Read the model definition and answer for the solid it produces. Units are mm, in the model's axes. A direction names the side the tool comes from. Coordinates: 2 decimals unless noted, no trailing zeros. Order: outer loops, then holes, each group sorted by start corner. A loop starts at its lowest first (then second) coordinate and runs counter-clockwise, first axis right, second up. Notation, with made-up numbers: (6, 84.5) - (14, 84.5) arc R27 ccw to (14, 122.5) - close; hole circle Ø4 at (75.25, 56.25). An arc over 180 degrees is marked (long way). Write item = value, one per line.
from build123d import *

# Parameters (mm, degrees)
CUT_EXTRUDE_1_DEPTH      = 170.966173207
CUT_EXTRUDE_1_DEPTH_BACK = 33


with BuildPart() as part:
    # 草图1 → 旋转1 (revolve)
    with BuildSketch(Plane(origin=(0, 0, 0), x_dir=(0, 0, -1), z_dir=(1, 0, 0)), mode=Mode.PRIVATE) as revolve_1_sk:
        with BuildLine():
            Line((-34.6, 0), (-34.6, 35))
            Line((-34.6, 35), (-22, 50))
            Line((-22, 50), (-22, 70))
            Line((-22, 70), (-21, 70))
            Line((-21, 70), (-21, 76))
            ThreePointArc((-21, 76), (0, 86.5), (21, 76))
            Line((21, 76), (21, 70))
            Line((21, 70), (22, 70))
            Line((22, 70), (22, 50))
            Line((22, 50), (34.6, 35))
            Line((34.6, 35), (34.6, 25))
            Line((34.6, 25), (40.4, 19.2))
            Line((40.4, 19.2), (40.4, 12))
            Line((40.4, 12), (45.4, 12))
            Line((45.4, 12), (45.4, 14))
            Line((45.4, 14), (48.4, 14))
            Line((48.4, 14), (48.4, 16))
            Line((48.4, 16), (50.4, 16))
            Line((50.4, 16), (50.4, 8))
            Line((50.4, 8), (83.4, 8))
            Line((83.4, 8), (83.4, 1.5))
            Line((83.4, 1.5), (88.4, 1.5))
            Line((88.4, 1.5), (88.4, 0))
            Line((88.4, 0), (-34.6, 0))
        make_face()
    revolve(revolve_1_sk.sketch.rotate(Axis((0, 0, 0), (0, 0, -1)), 90), axis=Axis((0, 0, 0), (0, 0, -1)))

    # 草图2 → 切除-拉伸1 (cut, two sides: drawn at the far end of the back side and taken through both)
    with BuildSketch(Plane(origin=(0, 0, -83.4), x_dir=(-1, 0, 0), z_dir=(0, 0, -1)).offset(-CUT_EXTRUDE_1_DEPTH_BACK)):
        with BuildLine():
            Line((-5.291502622, 6), (5.291502622, 6))
            ThreePointArc((5.291502622, 6), (0, 8), (-5.291502622, 6))
        make_face()
        with BuildLine():
            Line((-5.291502622, -6), (5.291502622, -6))
            ThreePointArc((5.291502622, -6), (0, -8), (-5.291502622, -6))
        make_face()
    extrude(amount=CUT_EXTRUDE_1_DEPTH + CUT_EXTRUDE_1_DEPTH_BACK, mode=Mode.SUBTRACT)


solid = part.part
1) The part is cut by section A-A (z = -7). Determine the outline of the cut face in (x, y), and give its area (3 significant figures).
Returned:
outline = circle Ø171.1 at (0, 0)
area = 23,000 mm^2
2) For faces 1 (the face through (8, 0, -67)), 2 (the face through (-15.175, 68.335, -21.507)), 3 (the face through (6.3, -10.4, -45.4)), 4 (the face through (0, 6, -67)), 5 (the face through (48, -17, 22)), determine the directions among +Z, -Z, +X, -X, +Y, -Y from which every point of the face is accessible in a straight line to the end or side of a thin tool.
Returned:
face_1 = -Z, +X
face_2 = -Z
face_3 = none
face_4 = -Z, +X, -X, +Y
face_5 = +Z
3) Determine the mould class of faces 6 (the face through (-8, 0, -67)), 7 (the face through (33, 62, -21)), 8 (the face through (0, 13, -40.4)) for opening direction Z: pulls with the +Z half, pulls with the -Z half, needs draft (parallel to the pull), parting line crosses it, or undercut.
Returned:
face_6 = needs draft
face_7 = pulls with the -Z half
face_8 = undercut
4) Flat-ended cylindrical pins translate along their axes: pin 1 Ø11.5 at (x, z) = (-2.5, -69) entering from -Y; pin 2 Ø2 at (y, z) = (-13.5, -7.5) entering from -X; pin 3 Ø6 at (x, z) = (-44.5, 7) entering from -Y. Find the tip coordinate at first contact, or state that the pin passes through.
Returned:
pin_1 = -6
pin_2 = -84.66
pin_3 = -75.02
5) Straight lines are drawn through the part: line 1 along X through (y, z) = (-34, 23); line 2 along Z through (x, y) = (38, 39.5); line 3 along Z through (x, y) = (-11, 33). For each, find the intervals that lie inside material, in ascending order. Write a range as from..to.
Returned:
line_1 = -35.02..35.02
line_2 = -22..22
line_3 = -34.6..34.6
